Can you work these out from the model? Positions are in its coordinate system, mm. Face numbers are marked on the shaded views. Coordinates: 2 decimals unless noted, no trailing zeros. Order: outer loops, then holes, each group sorted by start corner. A loop starts at its lowest first (then second) coordinate and runs counter-clockwise, first axis right, second up. Notation, with made-up numbers: (62, 38.5) -> (92, 38.5) arc R30 ccw to (92, 61.5) -> close; hole circle Ø3 at (40.5, 84.25). An arc over 180 degrees is marked (long way). Answer as CSV lines item,"result".
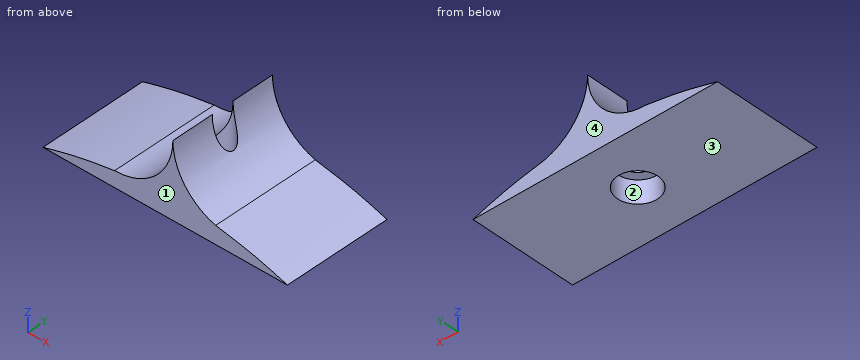
from build123d import *

# Parameters (mm, degrees)
F1_DEPTH = 12
F2_R     = 1.25
F3_DEPTH = 25
F2_R_2   = 2.25
F4_DEPTH = 2.5


with BuildPart() as f1:
    # F0 (on Front) → F1 (new body)
    with BuildSketch(Plane.XZ):
        with BuildLine():
            ThreePointArc((-15.0881102346, 0), (-16.991298859, -4.5955766968), (-21.5863641351, -6.4999997655))
            Line((-21.5863641351, -6.4999997655), (-21.5863641351, -8.2499998827))
            Line((-21.5863641351, -8.2499998827), (-10.3100242913, -8.2499998827))
            Line((-10.3100242913, -8.2499998827), (-10.3100242913, -6.2677756805))
            ThreePointArc((-10.3100242913, -6.2677756805), (-13.7573675008, -3.9406572188), (-15.0881102346, 0))
        make_face()
        with BuildLine():
            Line((-21.5863641351, -8.2499998827), (-21.5863641351, -6.4999997655))
            add(Edge.make_bspline(
                [(-21.5863641351, -6.4999997655), (-22.9185539989, -6.7095944516), (-25.5951490164, -7.1307056669), (-28.238998845, -7.875768386), (-29.566956684, -8.2499998827)],
                knots=[0, 0, 0, 0, 0.4977181288, 1, 1, 1, 1], degree=3))
            Line((-29.566956684, -8.2499998827), (-21.5863641351, -8.2499998827))
        make_face()
        with BuildLine():
            add(Edge.make_bspline(
                [(-10.3100242913, -6.2677756805), (-8.8950325252, -6.524315434), (-6.1143970315, -7.0284480808), (-3.563055622, -7.847662156), (-2.3100242913, -8.2499998827)],
                knots=[0, 0, 0, 0, 0.508873518, 1, 1, 1, 1], degree=3))
            Line((-10.3100242913, -6.2677756805), (-10.3100242913, -8.2499998827))
            Line((-10.3100242913, -8.2499998827), (-2.3100242913, -8.2499998827))
        make_face()
    extrude(amount=F1_DEPTH)

    # F2 (on face) → F3 (cut)
    with BuildSketch(Plane(origin=(0, 0, -8.2499998827), x_dir=(1, 0, 0), z_dir=(0, 0, -1))):
        with Locations((-15.1280872524, 5.9963222593)):
            Circle(F2_R)
    extrude(amount=-F3_DEPTH, mode=Mode.SUBTRACT)

    # F2 (on face) → F4 (cut)
    with BuildSketch(Plane(origin=(0, 0, -8.2499998827), x_dir=(1, 0, 0), z_dir=(0, 0, -1))):
        with Locations((-15.1280872524, 5.9963222593)):
            Circle(F2_R_2)
        with Locations((-15.1280872524, 5.9963222593)):
            Circle(F2_R, mode=Mode.SUBTRACT)
    extrude(amount=-F4_DEPTH, mode=Mode.SUBTRACT)


solid = f1.part
Q1. Imagine slicing it at A-A (z = -1). List the corners of the cut face in (x, y) for me.
Solution:
outline,"(-15.17, -12) -> (-15.01, -12) -> (-15.01, -7.24) arc R1.25 cw to (-15.17, -7.25) -> close; (-15.17, -4.75) arc R1.25 cw to (-15.01, -4.75) -> (-15.01, 0) -> (-15.17, 0) -> close"
Q2. Imagine slicing it at D-D (x = -10.75). List the corners of the cut face in (y, z) for me.
Solution:
outline,"(-12, -8.25) -> (0, -8.25) -> (0, -6.13) -> (-12, -6.13) -> close"
Q3. Imagine slicing it at B-B (x = -17). List the corners of the cut face in (y, z) for me.
Solution:
outline,"(-12, -8.25) -> (-7.24, -8.25) -> (-7.24, -5.75) -> (-4.75, -5.75) -> (-4.75, -8.25) -> (0, -8.25) -> (0, -4.6) -> (-12, -4.6) -> close"
Q4. For P1, Ø4, axis at x = -25.5, y = -3.5, coming from the +Z side; P2, Ø3, axis at y = -8.5, z = -2, coming from the -X side; P3, Ø1, axis at y = -7, z = -2, coming from the +X side, each with a flat end and sliding along its axis, tell me the tip position at first contact or that it passes through.
Solution:
P1,"z = -6.81"
P2,"x = -16.11"
P3,"x = -14.59"
Q5. Imagine slicing it at C-C (z = -3). List the corners of the cut face in (x, y) for me, and give its area (3 significant figures).
Solution:
outline,"(-15.82, -12) -> (-14.35, -12) -> (-14.35, -6.98) arc R1.25 cw to (-15.82, -7.04) -> close; (-15.82, -4.96) arc R1.25 cw to (-14.35, -5.01) -> (-14.35, 0) -> (-15.82, 0) -> close"
area,"14.2 mm2"
Q6. If I drill on line 1 (X direction, y = -10.5, z = -2.5); line 2 (X direction, y = -4.5, z = -4.75); line 3 (Z direction, x = -26.25, y = -6), over which ranges is the centre line in solid material (lowest first)?
Solution:
line 1,"-15.59 to -14.59"
line 2,"-17.15 to -13.03"
line 3,"-8.25 to -7.36"
Q7. We'd pull the mould along Y, two halves only. Please class the marked faces 1, 2, 3 and 4: pulls with the +Y half, pulls with the -Y half, needs draft (parallel to the pull), parting line crosses it, or undercut.
Solution:
face 1,"pulls with the -Y half"
face 2,"undercut"
face 3,"needs draft"
face 4,"pulls with the +Y half"
